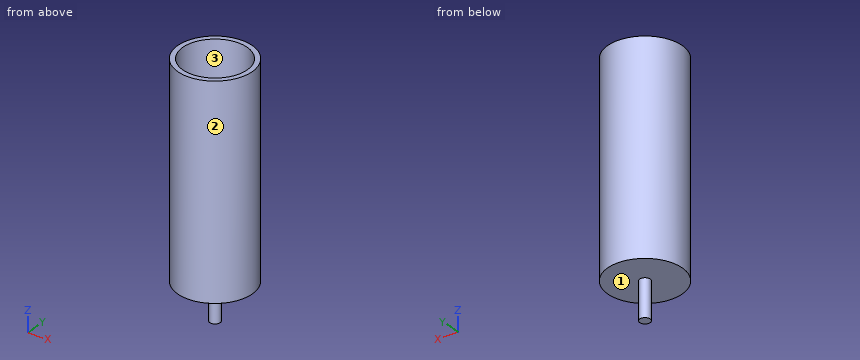
from build123d import *

# Parameters (mm, degrees)
SKETCH1_R           = 35
BOSS_EXTRUDE1_DEPTH = 195.58
SKETCH2_R           = 5
BOSS_EXTRUDE2_DEPTH = 35.052
SKETCH5_R           = 30.25
CUT_EXTRUDE1_DEPTH  = 152.4


with BuildPart() as part:
    # Sketch1 → Boss-Extrude1 (new body)
    with BuildSketch(Plane.XY):
        Circle(SKETCH1_R)
    extrude(amount=-BOSS_EXTRUDE1_DEPTH)

    # Sketch2 → Boss-Extrude2 (add)
    with BuildSketch(Plane(origin=(0, 0, -195.58), x_dir=(-1, 0, 0), z_dir=(0, 0, -1))):
        with Locations(Location((0, 0, 0), (0, 0, 180))):
            Circle(SKETCH2_R)
    extrude(amount=BOSS_EXTRUDE2_DEPTH)

    # Sketch5 → Cut-Extrude1 (cut)
    with BuildSketch(Plane.XY):
        Circle(SKETCH5_R)
    extrude(amount=-CUT_EXTRUDE1_DEPTH, mode=Mode.SUBTRACT)


solid = part.part
Build history of the part. All positions in model axes, mm. Face numbers are marked on the shaded views. Give positions to 0.01 mm unless a question says otherwise; leave off trailing zeros. Order: outer loops, then holes, each group sorted by start corner. A loop starts at its lowest first (then second) coordinate and runs counter-clockwise, first axis right, second up. Notation, with made-up numbers: M 79,51 L 132,51 A16 ccw 132,73 Z; hole C 26.5,8 d10. An arc over 180 degrees is marked long. Put each result on its own line as item: value.
Item 1: Flat gauge pins, fed straight in: pin 1 Ø8 at (x, y) = (-13.5, -17) entering from +Z; pin 2 Ø10 at (x, z) = (-6, -30) entering from +Y; pin 3 Ø10 at (x, y) = (-8, -25) entering from -Z. Where does each tip first touch, or does it go through?
From the geometry:
pin 1: stops at z = -152.4
pin 2: stops at y = 34.99
pin 3: stops at z = -195.58
Item 2: Slice it at A-A, the plane y = 0. Write the cut outline in (x, z), plus the area to 3 significant figures.
From the geometry:
outline: M -35,-195.58 L -5,-195.58 L -5,-230.63 L 5,-230.63 L 5,-195.58 L 35,-195.58 L 35,0 L 30.25,0 L 30.25,-152.4 L -30.25,-152.4 L -30.25,0 L -35,0 Z
area: 4,820 mm2
Item 3: Slice it at D-D, the plane y = -22. Write the cut outline in (x, z), plus the area to 3 significant figures.
From the geometry:
outline: M -27.22,-195.58 L 27.22,-195.58 L 27.22,0 L 20.76,0 L 20.76,-152.4 L -20.76,-152.4 L -20.76,0 L -27.22,0 Z
area: 4,320 mm2
Item 4: Slice it at B-B, the plane z = -111. Write the cut outline in (x, y), plus the area to 3 significant figures.
From the geometry:
outline: C 0,0 d70; hole C 0,0 d60.5
area: 974 mm2
Item 5: Two-plate mould, pull along X, no slides. Class the marked faces 1, 2 and 3: +X half, -X half, draft (parallel to the pull), parting line (faces both ways), or undercut.
From the geometry:
face 1: draft
face 2: parting line
face 3: undercut
Item 6: Probe line 1 (Y direction, x = 0, z = -60); line 2 (Z direction, x = -21, y = -27); line 3 (Z direction, x = -3, y = 17.5). List the from-to ranges inside material, lowest first. Write a range as [from, to].
From the geometry:
line 1: y = [-35, -30.25], [30.25, 35]
line 2: z = [-195.58, 0]
line 3: z = [-195.58, -152.4]
